```python
from build123d import *

# Parameters (mm, degrees)
SKETCH_R            = 25
PAD_DEPTH           = 8
PAD001_DEPTH        = 10
CHAMFER_SIZE        = 2
HOLE_D              = 5.5
HOLE_DEPTH          = 25
HOLE_CSINK_D        = 12.7
HOLE_CSINK_ANGLE    = 90
HOLE001_D           = 3.4
HOLE001_DEPTH       = 25
HOLE001_CSINK_D     = 6.7
HOLE001_CSINK_ANGLE = 90
CHAMFER001_SIZE     = 2


with BuildPart() as part:
    # Sketch → Pad (new body)
    with BuildSketch(Plane.XY):
        Circle(SKETCH_R)
    extrude(amount=PAD_DEPTH)

    # Sketch001 (on Face3 of Pad) → Pad001 (join)
    with BuildSketch(Plane.XY.offset(8)):
        with BuildLine():
            ThreePointArc((0, 25), (-25, 0), (0, -25))
            Line((150.871382, -17.478292), (0, -25))
            ThreePointArc((150.871382, -17.478292), (167.5, 0), (150.871382, 17.478292))
            Line((0, 25), (150.871382, 17.478292))
        make_face()
    extrude(amount=PAD001_DEPTH)

    # Chamfer
    chamfer_edges = [part.edges().sort_by_distance(p)[0] for p in [
        (75.435691, -21.239146, 18),
    ]]
    chamfer(chamfer_edges, length=CHAMFER_SIZE)

    # Hole
    with Locations(Plane.XY.offset(18)):
        with Locations((-12.5, 12.5), (12.5, 12.5), (12.5, -12.5), (-12.5, -12.5)):
            CounterSinkHole(HOLE_D / 2, HOLE_CSINK_D / 2, depth=HOLE_DEPTH, counter_sink_angle=HOLE_CSINK_ANGLE)

    # Hole001
    with Locations(Plane.XY.offset(18)):
        with Locations((142.5, 7.5), (157.5, 7.5), (157.5, -7.5), (142.5, -7.5), (150, 0)):
            CounterSinkHole(HOLE001_D / 2, HOLE001_CSINK_D / 2, depth=HOLE001_DEPTH, counter_sink_angle=HOLE001_CSINK_ANGLE)

    # Chamfer001
    chamfer001_edges = [part.edges().sort_by_distance(p)[0] for p in [
        (-25, 0, 0),
    ]]
    chamfer(chamfer001_edges, length=CHAMFER001_SIZE)


solid = part.part
```
Verification items for the finished model (mm, model axes). Round coordinates to 2 decimals unless told otherwise and drop trailing zeros. Write each loop counter-clockwise with the first axis right and the second up, starting at its lowest first coordinate (ties: lowest second). Pieces come first, ordered by that corner, then holes.
1. Section check A-A on y = 0. Enter the section's corners in (x, z).
2. Draft check along X on faces 1 (the conical face through (-23.314, -0.513, 17.681)), 2 (the flat face through (0, 0, 0)), 3 (the cylindrical face through (9.88, -11.67, 7.1)). Enter one of: +X half, -X half, draft (parallel to the pull), parting line (faces both ways), or undercut.
3. Section check B-B on z = 10. State how many separate pieces and enclosed holes the cut face has, plus the area to 3 significant figures.
4. Gauge pin test, flat ends, axial feed: P1, Ø4.5, axis at x = 12.5, y = -12.5, coming from the +Z side; P2, Ø4, axis at x = 2.5, z = 13.5, coming from the +Y side; P3, Ø10, axis at y = 8.5, z = 3.5, coming from the +X side; P4, Ø1.5, axis at y = 2.5, z = 12, coming from the +X side. Record the tip position at first contact, or that the pin passes through.
5. Scan lines: L1, parallel to Y at x = 157.5, z = 11; L2, parallel to X at y = 0, z = 10.25; L3, parallel to Y at x = 12.5, z = 8.75. Record each from-to range of solid material in increasing order.
6. Section check D-D on x = 40.5. Enter the section's corners in (y, z), plus the area to 3 significant figures.
7. Section check C-C on x = 142.5. Enter the section's corners in (y, z), plus the area to 3 significant figures.
Answer:
1. outline: (-25, 2) - (-23, 0) - (23, 0) - (25, 2) - (25, 8) - (148.3, 8) - (148.3, 16.35) - (146.65, 18) - (-23, 18) - (-25, 16) - close; (151.7, 8) - (167.5, 8) - (167.5, 16) - (165.5, 18) - (153.35, 18) - (151.7, 16.35) - close
2. face 1: -X half
2. face 2: draft
2. face 3: undercut
3. separate pieces: 1
3. enclosed holes: 9
3. area: 7,700 mm2
4. P1: passes through
4. P2: stops at y = 24.98
4. P3: stops at x = 166.32
4. P4: stops at x = 167.41
5. L1: y = -15.81 to -9.2, -5.8 to 5.8, 9.2 to 15.81
5. L2: x = -25 to 148.3, 151.7 to 167.5
5. L3: y = -24.38 to -15.25, -9.75 to 9.75, 15.25 to 24.38
6. outline: (-22.98, 8) - (22.98, 8) - (22.98, 16) - (20.98, 18) - (-20.98, 18) - (-22.98, 16) - close
6. area: 456 mm2
7. outline: (-17.9, 8) - (-9.2, 8) - (-9.2, 16.35) - (-10.85, 18) - (-15.89, 18) - (-17.9, 16) - close; (-5.8, 8) - (5.8, 8) - (5.8, 16.35) - (4.15, 18) - (-4.15, 18) - (-5.8, 16.35) - close; (9.2, 8) - (17.9, 8) - (17.9, 16) - (15.89, 18) - (10.85, 18) - (9.2, 16.35) - close
7. area: 280 mm2
